```python
from build123d import *

# Parameters (mm, degrees)
SKETCH1_W           = 33
SKETCH1_H           = 8
BOSS_EXTRUDE1_DEPTH = 3
BOSS_EXTRUDE2_DEPTH = 16.5
BOSS_EXTRUDE3_DEPTH = 13


with BuildPart() as part:
    # Sketch1 → Boss-Extrude1 (new body)
    with BuildSketch(Plane(origin=(0, 0, 0), x_dir=(1, 0, 0), z_dir=(0, 1, 0))):
        with Locations((41.871824735, 0)):
            Rectangle(SKETCH1_W, SKETCH1_H)
    extrude(amount=BOSS_EXTRUDE1_DEPTH)

    # Sketch1_6 → Boss-Extrude2 (add)
    with BuildSketch(Plane(origin=(0, 0, 0), x_dir=(1, 0, 0), z_dir=(0, 1, 0))):
        with BuildLine():
            Line((58.371824735, 4), (58.371824735, 0))
            Line((58.371824735, 0), (65.371824735, 0))
            ThreePointArc((65.371824735, 0), (65.041534478, 7.03096345), (64.053572815, 14))
            Line((64.053572815, 14), (43.371824735, 14))
            Line((43.371824735, 14), (43.371824735, 4))
            Line((43.371824735, 4), (58.371824735, 4))
        make_face()
        with BuildLine():
            Line((65.371824735, 0), (58.371824735, 0))
            Line((58.371824735, 0), (58.371824735, -4))
            Line((58.371824735, -4), (43.371824735, -4))
            Line((43.371824735, -4), (43.371824735, -14))
            Line((43.371824735, -14), (64.053572815, -14))
            ThreePointArc((64.053572815, -14), (65.041534478, -7.03096345), (65.371824735, 0))
        make_face()
    extrude(amount=BOSS_EXTRUDE2_DEPTH)

    # Sketch1_7 → Boss-Extrude3 (add)
    with BuildSketch(Plane(origin=(0, 0, 0), x_dir=(1, 0, 0), z_dir=(0, 1, 0))):
        with BuildLine():
            Line((25.371824735, -4), (25.371824735, 4))
            Line((25.371824735, 4), (43.371824735, 4))
            Line((43.371824735, 4), (43.371824735, 14))
            Line((43.371824735, 14), (29.371824735, 14))
            ThreePointArc((29.371824735, 14), (15.371824735, 0), (29.371824735, -14))
            Line((29.371824735, -14), (43.371824735, -14))
            Line((43.371824735, -14), (43.371824735, -4))
            Line((43.371824735, -4), (25.371824735, -4))
        make_face()
    extrude(amount=BOSS_EXTRUDE3_DEPTH)


solid = part.part
```
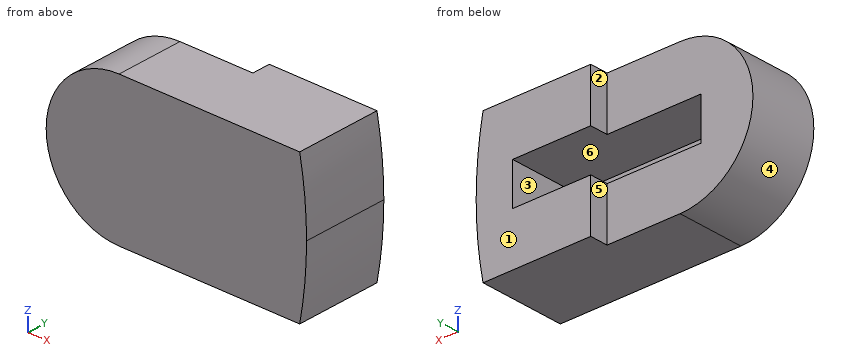
Here's how the part is built. I have some questions about the finished solid (model axes, mm). Face numbers are marked on the shaded views. A direction names the side the tool comes from. Round coordinates to 2 decimals unless told otherwise and drop trailing zeros. Loops run counter-clockwise (first coordinate to the right, second up) from the corner with the lowest first, then second, coordinate; pieces in that order, holes last. Notation, with made-up numbers: (40, 53) -> (70, 53) arc R22 ccw to (70, 73) -> close; hole circle Ø1 at (-33.75, 67.25). An arc over 180 degrees is marked (long way). Answer as CSV lines item,"result".
1. If we section it at B-B on x = 32: Please give me the cut outline in (y, z), plus the area to 3 significant figures.
Final values:
outline,"(0, -14) -> (13, -14) -> (13, -4) -> (3, -4) -> (3, 4) -> (13, 4) -> (13, 14) -> (0, 14) -> close"
area,"284 mm^2"
2. If I drill on L1, parallel to Z at x = 30.5, y = 4; L2, parallel to X at y = 8, z = -2.5; L3, parallel to Y at x = 42.5, z = 11.75, over which ranges is the centre line in solid material (lowest first)?
Final values:
L1,"z = -14 to -4, 4 to 14"
L2,"x = 15.6 to 25.37, 58.37 to 65.33"
L3,"y = 0 to 13"
3. For pin 1 (2 mm diameter, centred on x = 49, z = 0.5, fed in from +Y); pin 2 (1.5 mm diameter, centred on y = 4, z = 3, fed in from -X); pin 3 (4 mm diameter, centred on y = 4, z = -10, fed in from -X), each with a flat end and sliding along its axis, tell me the tip position at first contact or that it passes through.
Final values:
pin 1,"stops at y = 3"
pin 2,"stops at x = 15.55"
pin 3,"stops at x = 17.88"
4. Thinking about a two-plate mould opening in Z: for the marked faces 4, 5 and 6, which applies, released by +Z, released by -Z, zero draft, split by the parting line, or undercut?
Final values:
face 4,"split by the parting line"
face 5,"zero draft"
face 6,"undercut"
5. If we section it at C-C on z = -8.25: Please give me the cut outline in (x, y).
Final values:
outline,"(18.06, 0) -> (64.92, 0) -> (64.92, 16.5) -> (43.37, 16.5) -> (43.37, 13) -> (18.06, 13) -> close"
6. If we section it at A-A on y = 8: Please give me the cut outline in (x, z), plus the area to 3 significant figures.
Final values:
outline,"(29.37, -14) -> (64.05, -14) arc R75 ccw to (64.05, 14) -> (29.37, 14) arc R14 ccw to start; hole (25.37, -4) -> (58.37, -4) -> (58.37, 4) -> (25.37, 4) -> close"
area,"1,040 mm^2"
7. Which directions (+Z, -Z, +X, -X, +Y, -Y) give clear straight access to the entire face, cutting with the end or side of a thin tool? Please do the marked faces 1, 2 and 3.
Final values:
face 1,"+Z, -Z, +X, -X, +Y"
face 2,"+Z, -Z, -X, +Y"
face 3,"+Y"
8. If we section it at D-D on x = 48.5: Please give me the cut outline in (y, z), plus the area to 3 significant figures.
Final values:
outline,"(0, -14) -> (16.5, -14) -> (16.5, -4) -> (3, -4) -> (3, 4) -> (16.5, 4) -> (16.5, 14) -> (0, 14) -> close"
area,"354 mm^2"
